CAD build for the part. Positions are in the model's coordinates, mm. A direction names the side the tool comes from. Give positions to 0.01 mm unless a question says otherwise; leave off trailing zeros. Write each loop counter-clockwise with the first axis right and the second up, starting at its lowest first coordinate (ties: lowest second). Pieces come first, ordered by that corner, then holes. Notation, with made-up numbers: (6, 60) - (56, 60) arc R20 ccw to (56, 94) - close; hole circle Ø11 at (59.25, 64.25). An arc over 180 degrees is marked (long way). Answer as a JSON object with one key per item and string values.
from build123d import *

# Parameters (mm, degrees)
SKETCH1_R           = 15
BOSS_EXTRUDE1_DEPTH = 40
BOSS_EXTRUDE2_DEPTH = 20
BOSS_EXTRUDE3_START = -20
BOSS_EXTRUDE3_DEPTH = 20
SKETCH4_W           = 100
SKETCH4_H           = 50
BOSS_EXTRUDE4_DEPTH = 80
SKETCH5_R           = 60
BOSS_EXTRUDE5_DEPTH = 10
SKETCH6_R           = 15
CUT_EXTRUDE1_DEPTH  = 10
CUT_EXTRUDE2_DEPTH  = 90
CUT_EXTRUDE3_DEPTH  = 90
FILLET2_R           = 10


with BuildPart() as part:
    # Sketch1 → Boss-Extrude1 (new, symmetric)
    with BuildSketch(Plane.XY):
        Circle(SKETCH1_R)
    extrude(amount=BOSS_EXTRUDE1_DEPTH, both=True)

    # Sketch2 → Boss-Extrude2 (add)
    with BuildSketch(Plane.XY.offset(40)):
        with BuildLine():
            Line((50, 0), (50, -70))
            ThreePointArc((50, -70), (0, -120), (-50, -70))
            Line((-50, -70), (-50, 0))
            ThreePointArc((-50, 0), (0, 50), (50, 0))
        make_face()
    extrude(amount=-BOSS_EXTRUDE2_DEPTH)

    # Sketch3 → Boss-Extrude3 (add)
    with BuildSketch(Plane(origin=(0, 0, -40), x_dir=(-1, 0, 0), z_dir=(0, 0, -1)).offset(BOSS_EXTRUDE3_START)):
        with BuildLine():
            Line((50, 0), (50, -70))
            ThreePointArc((50, -70), (0, -120), (-50, -70))
            Line((-50, -70), (-50, 0))
            ThreePointArc((-50, 0), (0, 50), (50, 0))
        make_face()
    extrude(amount=BOSS_EXTRUDE3_DEPTH)

    # Sketch4 → Boss-Extrude4 (add)
    with BuildSketch(Plane(origin=(0, 0, -40), x_dir=(-1, 0, 0), z_dir=(0, 0, -1))):
        with Locations((0, -95)):
            Rectangle(SKETCH4_W, SKETCH4_H)
    extrude(amount=-BOSS_EXTRUDE4_DEPTH)

    # Sketch5 → Boss-Extrude5 (add)
    with BuildSketch(Plane.XZ.offset(120)):
        with Locations(Location((0, 0, 0), (0, 0, 41.810314896))):
            Circle(SKETCH5_R)
    extrude(amount=BOSS_EXTRUDE5_DEPTH)

    # Sketch6 → Cut-Extrude1 (cut)
    with BuildSketch(Plane.XZ.offset(130)):
        with Locations(Location((0, 0, 0), (0, 0, 270))):
            Circle(SKETCH6_R)
    extrude(amount=-CUT_EXTRUDE1_DEPTH, mode=Mode.SUBTRACT)

    # Sketch7 → Cut-Extrude2 (cut)
    with BuildSketch(Plane.XY.offset(40)):
        with BuildLine():
            Line((-50, -70), (-50, 0))
            ThreePointArc((-50, 0), (-35.502525317, -35), (-50, -70))
        make_face()
    extrude(amount=-CUT_EXTRUDE2_DEPTH, mode=Mode.SUBTRACT)

    # Sketch8 → Cut-Extrude3 (cut)
    with BuildSketch(Plane.XY.offset(40)):
        with BuildLine():
            Line((50, -70), (50, 0))
            ThreePointArc((50, 0), (35.502525317, -35), (50, -70))
        make_face()
    extrude(amount=-CUT_EXTRUDE3_DEPTH, mode=Mode.SUBTRACT)

    # Fillet2
    fillet2_edges = [part.edges().sort_by_distance(p)[0] for p in [
        (50, 0, -30),
        (-50, 0, -30),
        (-50, 0, 30),
        (50, 0, 30),
    ]]
    fillet(fillet2_edges, radius=FILLET2_R)


solid = part.part
(1) Flat gauge pins, fed straight in: P1, Ø6, axis at x = -26.5, y = -68.5, coming from the -Z side; P2, Ø10, axis at x = -10.5, y = -39.5, coming from the +Z side; P3, Ø1, axis at x = -34, z = -34, coming from the +Y side. Where does each tip first touch, or does it go through?
Answer key:
{"P1": "stops at z = -40", "P2": "stops at z = 40", "P3": "stops at y = 37.12"}
(2) Saw through at A-A, the plane x = 0. Give the cut face in (y, z).
Answer key:
{"outline": "(-130, -60) - (-120, -60) - (-120, -40) - (50, -40) - (50, -20) - (15, -20) - (15, 20) - (50, 20) - (50, 40) - (-120, 40) - (-120, 60) - (-130, 60) - (-130, 15) - (-120, 15) - (-120, -15) - (-130, -15) - close; hole (-70, -20) - (-15, -20) - (-15, 20) - (-70, 20) - close"}
(3) 3-axis set-ups, long thin cutter, end or side, ignore diameter. For faces 4 (the face through (1, -70, 0)), 5 (the face through (56.123, -124.93, -21.218)), 6 (the face through (49, -120, 38)), 7 (the face through (2, -120, -50)): which of +Z, -Z, +X, -X, +Y, -Y reach the whole face in a straight line?
Answer key:
{"face 4": "+X, -X", "face 5": "-Y", "face 6": "+Z, +X, -Y", "face 7": "-Z, +X, -X, +Y"}
(4) Pull direction Y, two halves, no side cores. Call faces 1 (the face through (1, -22, 20)), 2 (the face through (0, -120, 0)), 3 (the face through (1.03, 49.99, -29.86)): pulls with the +Y half, pulls with the -Y half, needs draft (parallel to the pull), parting line crosses it, or undercut.
Answer key:
{"face 1": "undercut", "face 2": "pulls with the -Y half", "face 3": "pulls with the +Y half"}
(5) Saw through at B-B, the plane z = 0. Give the cut face in (x, y), and give its area (3 significant figures).
Answer key:
{"outline": "(-60, -130) - (-15, -130) - (-15, -120) - (15, -120) - (15, -130) - (60, -130) - (60, -120) - (50, -120) - (50, -70) - (-50, -70) - (-50, -120) - (-60, -120) - close; circle Ø30 at (0, 0)", "area": "6,610 mm²"}
(6) Probe L1, parallel to X at y = -127.5, z = 0; L2, parallel to Z at x = -26.5, y = 6.5; L3, parallel to Y at x = 1, z = 2.5. List the from-to ranges inside material, lowest first. Write a range as [from, to].
Answer key:
{"L1": "x = [-60, -15], [15, 60]", "L2": "z = [-40, -20], [20, 40]", "L3": "y = [-120, -70], [-14.97, 14.97]"}
(7) Saw through at D-D, the plane y = -92. Give the cut face in (x, z).
Answer key:
{"outline": "(-50, -40) - (50, -40) - (50, 40) - (-50, 40) - close"}
(8) Saw through at C-C, the plane y = 39. Give the cut face in (x, z), and give its area (3 significant figures).
Answer key:
{"outline": "(-31.29, -40) - (31.29, -40) - (31.29, -20) - (-31.29, -20) - close; (-31.29, 20) - (31.29, 20) - (31.29, 40) - (-31.29, 40) - close", "area": "2,500 mm²"}
